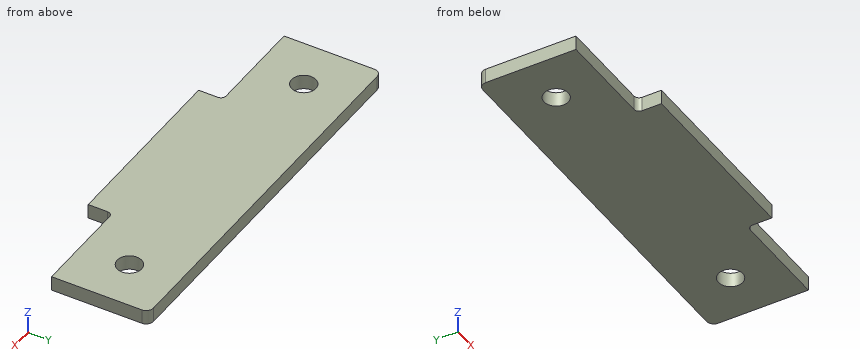
```python
from build123d import *

# Parameters (mm, degrees)
SKETCH_1_R      = 2.5
EXTRUDE_1_DEPTH = 3
FILLET_1_R      = 1.05
FILLET_2_R      = 1.5


with BuildPart() as part:
    # ｽｹｯﾁ1 → ﾎﾞｽ - 押し出し1 (new body)
    with BuildSketch(Plane.XY):
        Polygon((-19, 0), (19, 0), (19, 5), (40, 5), (40, 25), (-40, 25), (-40, 5), (-19, 5), align=None)
        with Locations((-30, 15)):
            Circle(SKETCH_1_R, mode=Mode.SUBTRACT)
        with Locations(Location((30, 15, 0), (0, 0, 180))):
            Circle(SKETCH_1_R, mode=Mode.SUBTRACT)
    extrude(amount=EXTRUDE_1_DEPTH)

    # ﾌｨﾚｯﾄ1
    fillet_1_edges = [part.edges().sort_by_distance(p)[0] for p in [
        (-19, 5, 1.5),
        (19, 5, 1.5),
    ]]
    fillet(fillet_1_edges, radius=FILLET_1_R)

    # ﾌｨﾚｯﾄ2
    fillet_2_edges = [part.edges().sort_by_distance(p)[0] for p in [
        (-40, 25, 1.5),
        (40, 25, 1.5),
    ]]
    fillet(fillet_2_edges, radius=FILLET_2_R)


solid = part.part
```
The listing builds one solid part. Answer for the finished solid, in the listing's coordinates (mm). Coordinates: 2 decimals unless noted, no trailing zeros. Write each loop counter-clockwise with the first axis right and the second up, starting at its lowest first coordinate (ties: lowest second). Pieces come first, ordered by that corner, then holes. Notation, with made-up numbers: (87, 4) - (111, 4) arc R21 cw to (111, 43) - close; hole circle Ø11 at (-35, -17). An arc over 180 degrees is marked (long way). Return JSON: item names as keys, results as strings. Group by question number.
Q1. The part is cut by section B-B on z = 0.5. Write down the section's boundary in (x, y).
Q2. Find the intervals of material crossed by line 1 along X through (y, z) = (16, 0.5); line 2 along Y through (x, z) = (30, 1.25); line 3 along X through (y, z) = (14.25, 0.6), in increasing order. Write a range as [from, to].
Q3. The part is cut by section A-A on x = -30. Write down the section's boundary in (y, z).
Q4. The part is cut by section D-D on x = 28.5. Write down the section's boundary in (y, z), and give its area (3 significant figures).
Q5. The part is cut by section C-C on y = 15. Write down the section's boundary in (x, z), and give its area (3 significant figures).
Q6. Flat-ended cylindrical pins translate along their axes: pin 1 Ø1.5 at (y, z) = (2.5, 2) entering from +X; pin 2 Ø4 at (x, y) = (-30, 15) entering from +Z; pin 3 Ø1.5 at (x, z) = (-33.5, 1) entering from -Y. Find the tip coordinate at first contact, or state that the pin passes through.
Evaluation:
{
 "1": {"outline": "(-40, 5) - (-20.05, 5) arc R1.05 cw to (-19, 3.95) - (-19, 0) - (19, 0) - (19, 3.95) arc R1.05 cw to (20.05, 5) - (40, 5) - (40, 23.5) arc R1.5 ccw to (38.5, 25) - (-38.5, 25) arc R1.5 ccw to (-40, 23.5) - close; hole circle Ø5 at (-30, 15); hole circle Ø5 at (30, 15)"},
 "2": {"line 1": "x = [-40, -32.29], [-27.71, 27.71], [32.29, 40]", "line 2": "y = [5, 12.5], [17.5, 25]", "line 3": "x = [-40, -32.38], [-27.62, 27.62], [32.38, 40]"},
 "3": {"outline": "(5, 0) - (12.5, 0) - (12.5, 3) - (5, 3) - close; (17.5, 0) - (25, 0) - (25, 3) - (17.5, 3) - close"},
 "4": {"outline": "(5, 0) - (13, 0) - (13, 3) - (5, 3) - close; (17, 0) - (25, 0) - (25, 3) - (17, 3) - close", "area": "48.0 mm2"},
 "5": {"outline": "(-40, 0) - (-32.5, 0) - (-32.5, 3) - (-40, 3) - close; (-27.5, 0) - (27.5, 0) - (27.5, 3) - (-27.5, 3) - close; (32.5, 0) - (40, 0) - (40, 3) - (32.5, 3) - close", "area": "210 mm2"},
 "6": {"pin 1": "stops at x = 19", "pin 2": "passes through", "pin 3": "stops at y = 5"}
}
